Input: dimensioned drawing with shaded views. Units: mm. Origin: part minimum x, y, z. Coordinates: 2 decimals unless noted, no trailing zeros. Loops run counter-clockwise (first coordinate to the right, second up) from the corner with the lowest first, then second, coordinate; pieces in that order, holes last. Notation, with made-up numbers: (-33.5, 1.5) -> (-20.5, 1.5) arc R12 cw to (-20.5, 7.5) -> close; hole circle Ø11 at (12, 83.5). An arc over 180 degrees is marked (long way). Answer as CSV lines item,"result".
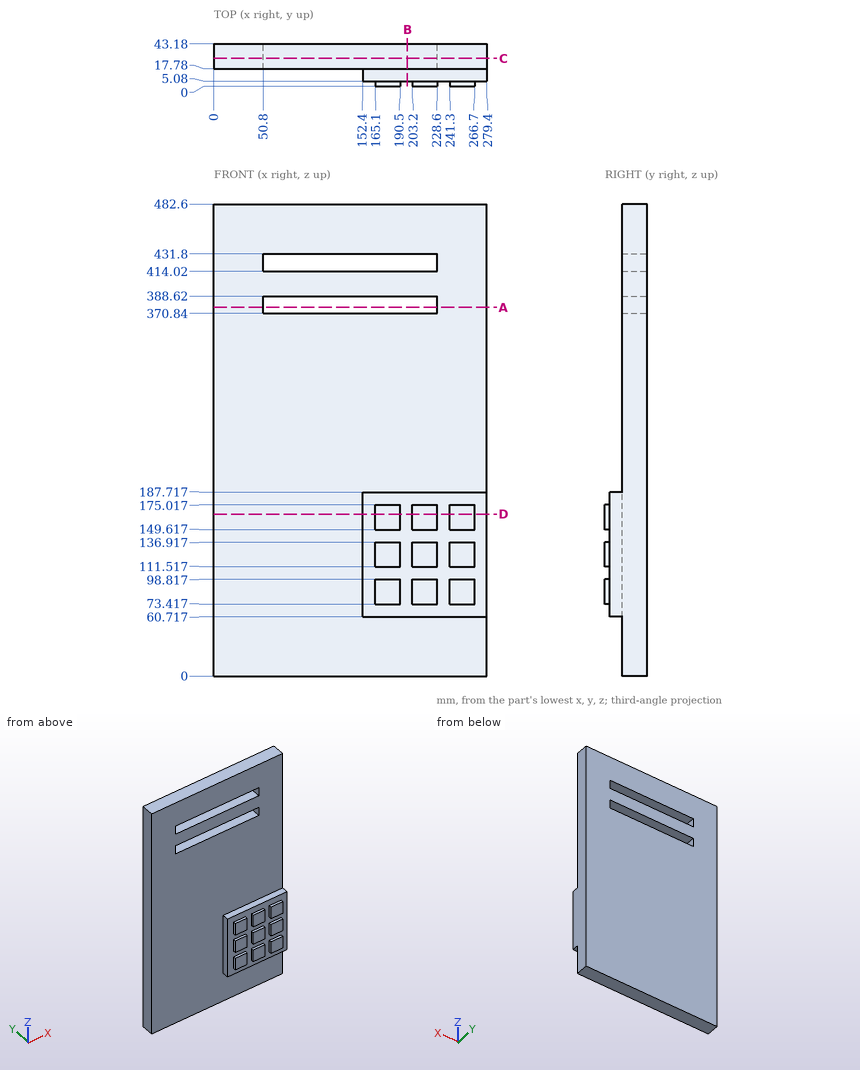
(1) Cut plane D-D (z = 165.5). Return the cut outline in (x, y).
Computed values:
outline,"(0, 17.78) -> (152.4, 17.78) -> (152.4, 5.08) -> (165.1, 5.08) -> (165.1, 0) -> (190.5, 0) -> (190.5, 5.08) -> (203.2, 5.08) -> (203.2, 0) -> (228.6, 0) -> (228.6, 5.08) -> (241.3, 5.08) -> (241.3, 0) -> (266.7, 0) -> (266.7, 5.08) -> (279.4, 5.08) -> (279.4, 43.18) -> (0, 43.18) -> close"
(2) Cut plane C-C (y = 28.5). Return the cut outline in (x, z), then the cut area to 3 significant figures.
Computed values:
outline,"(0, 0) -> (279.4, 0) -> (279.4, 482.6) -> (0, 482.6) -> close; hole (50.8, 370.84) -> (228.6, 370.84) -> (228.6, 388.62) -> (50.8, 388.62) -> close; hole (50.8, 414.02) -> (228.6, 414.02) -> (228.6, 431.8) -> (50.8, 431.8) -> close"
area,"129,000 mm^2"
(3) Cut plane B-B (x = 198). Return the cut outline in (y, z), then the cut area to 3 significant figures.
Computed values:
outline,"(5.08, 60.72) -> (17.78, 60.72) -> (17.78, 0) -> (43.18, 0) -> (43.18, 370.84) -> (17.78, 370.84) -> (17.78, 187.72) -> (5.08, 187.72) -> close; (17.78, 388.62) -> (43.18, 388.62) -> (43.18, 414.02) -> (17.78, 414.02) -> close; (17.78, 431.8) -> (43.18, 431.8) -> (43.18, 482.6) -> (17.78, 482.6) -> close"
area,"13,000 mm^2"
(4) Pin query (flat end, axial travel): pin 1 Ø10 at (y, z) = (8, 292) entering from +X; pin 2 Ø1.5 at (y, z) = (3.5, 130.5) entering from -X; pin 3 Ø2.5 at (x, y) = (214, 2) entering from +Z; pin 4 Ø12 at (x, z) = (132, 321.5) entering from -Y. Return the tip coordinate at first contact, or that it passes through.
Computed values:
pin 1,"through"
pin 2,"x = 165.1"
pin 3,"z = 175.02"
pin 4,"y = 17.78"
(5) Cut plane A-A (z = 377). Return the cut outline in (x, y), then the cut area to 3 significant figures.
Computed values:
outline,"(0, 17.78) -> (50.8, 17.78) -> (50.8, 43.18) -> (0, 43.18) -> close; (228.6, 17.78) -> (279.4, 17.78) -> (279.4, 43.18) -> (228.6, 43.18) -> close"
area,"2,580 mm^2"
(6) Material intervals for L1, parallel to Z at x = 176, y = 36; L2, parallel to Y at x = 61, z = 90; L3, parallel to X at y = 11.5, z = 95, sorted ascending. Write a range as [from, to].
Computed values:
L1,"[0, 370.84], [388.62, 414.02], [431.8, 482.6]"
L2,"[17.78, 43.18]"
L3,"[152.4, 279.4]"
